Could you check a few things on this model? Use its own coordinates, in mm. A direction names the side the tool comes from. Coordinates: 2 decimals unless noted, no trailing zeros. Write each loop counter-clockwise with the first axis right and the second up, starting at its lowest first coordinate (ties: lowest second). Pieces come first, ordered by that corner, then holes.
```python
from build123d import *

# Parameters (mm, degrees)
F0_W     = 88.9
F0_H     = 63.5
F0_W_2   = 64.688936
F0_H_2   = 39.437553
F1_DEPTH = 25.4
F2_W     = 64.972658
F2_H     = 38.870107
F3_DEPTH = 7.62
F5_DEPTH = 19.05
F7_DEPTH = 19.05


with BuildPart() as f1:
    # F0 (on Top) → F1 (new body)
    with BuildSketch(Plane.XY):
        with Locations((-7.991541, 0.256701)):
            Rectangle(F0_W, F0_H)
        with Locations((-8.937288, 0.425585)):
            Rectangle(F0_W_2, F0_H_2, mode=Mode.SUBTRACT)
    extrude(amount=F1_DEPTH)

    # F2 (on Top) → F3 (join)
    with BuildSketch(Plane.XY):
        with Locations((-9.079149, 0.425584)):
            Rectangle(F2_W, F2_H)
    extrude(amount=F3_DEPTH)

    # F4 (on Top) → F5 (join)
    with BuildSketch(Plane.XY):
        Polygon((-14.895479, 10.781489), (-34.756117, 10.781489), (-34.756117, 2.269787), (-28.797926, 2.269787), (-28.797926, -13.902447), (-21.421118, -13.902447), (-21.421118, 2.269787), (-14.895479, 2.269787), align=None)
    extrude(amount=F5_DEPTH)

    # F6 (on Top) → F7 (join)
    with BuildSketch(Plane.XY):
        Polygon((2.127926, 10.497767), (-3.830266, 10.497767), (-3.830266, -13.335001), (14.895479, -13.335001), (14.895479, -6.241915), (2.127926, -6.241915), align=None)
    extrude(amount=F7_DEPTH)


solid = f1.part
```
Item 1: I want a section at D-D, the plane z = 23.25. List the corners of the cut face in (x, y) for me.
Item 2: I want a section at B-B, the plane x = -20.5. List the corners of the cut face in (y, z) for me.
Item 3: Which directions (+Z, -Z, +X, -X, +Y, -Y) give clear straight access to the entire face, cutting with the end or side of a thin tool? Please do faces 1 (the flat face through (-52.442, 0, 13)), 2 (the flat face through (5, -13.335, 13)), 3 (the flat face through (-9, -19.293, 13)).
Item 4: I want a section at A-A, the plane z = 13.5. List the corners of the cut face in (x, y) for me (3 decimals), then the cut area to 3 significant figures.
Item 5: If we mould it in two halves opening along Y, with no side actions, what happens to faces 4 (the flat face through (-9, -31.493, 13)), 5 (the flat face through (-9, 1, 0)), 6 (the flat face through (-28.798, -6, 13))? For each: released by +Y, released by -Y, zero draft, split by the parting line, or undercut.
Item 6: If I drill on line 1 along Y through (x, z) = (-23.5, 2.25); line 2 along X through (y, z) = (7, 9.5); line 3 along Y through (x, z) = (-29, 13), over which ranges is the centre line in solid material (lowest first)?
Item 7: Will these pins go through, and if not, where does the flat tip stop? pin 1 Ø3 at (x, y) = (-15, 8.5) entering from +Z; pin 2 Ø1 at (x, y) = (-40.5, 8.5) entering from +Z.
Item 8: I want a section at C-C, the plane y = 9. List the corners of the cut face in (x, z) for me, then the cut area to 3 significant figures.
Taken from the geometry:
1. outline: (-52.44, -31.49) - (36.46, -31.49) - (36.46, 32.01) - (-52.44, 32.01) - close; hole (-41.28, -19.29) - (23.41, -19.29) - (23.41, 20.14) - (-41.28, 20.14) - close
2. outline: (-31.49, 0) - (-19.29, 0) - (-19.29, 25.4) - (-31.49, 25.4) - close; (-19.01, 0) - (19.86, 0) - (19.86, 7.62) - (10.78, 7.62) - (10.78, 19.05) - (2.27, 19.05) - (2.27, 7.62) - (-19.01, 7.62) - close; (20.14, 0) - (32.01, 0) - (32.01, 25.4) - (20.14, 25.4) - close
3. face 1: +Z, -Z, -X, +Y, -Y
3. face 2: +Z
3. face 3: +Z, -Z
4. outline: (-52.442, -31.493) - (36.458, -31.493) - (36.458, 32.007) - (-52.442, 32.007) - close; (-34.756, 2.27) - (-28.798, 2.27) - (-28.798, -13.902) - (-21.421, -13.902) - (-21.421, 2.27) - (-14.895, 2.27) - (-14.895, 10.781) - (-34.756, 10.781) - close; (-3.83, -13.335) - (14.895, -13.335) - (14.895, -6.242) - (2.128, -6.242) - (2.128, 10.498) - (-3.83, 10.498) - close; hole (-41.282, -19.293) - (23.407, -19.293) - (23.407, 20.144) - (-41.282, 20.144) - close
4. area: 3,610 mm2
5. face 4: released by -Y
5. face 5: zero draft
5. face 6: undercut
6. line 1: y = -31.49 to -19.29, -19.01 to 19.86, 20.14 to 32.01
6. line 2: x = -52.44 to -41.28, -34.76 to -14.9, -3.83 to 2.13, 23.41 to 36.46
6. line 3: y = -31.49 to -19.29, 2.27 to 10.78, 20.14 to 32.01
7. pin 1: stops at z = 19.05
7. pin 2: stops at z = 7.62
8. outline: (-52.44, 0) - (36.46, 0) - (36.46, 25.4) - (23.41, 25.4) - (23.41, 7.62) - (2.13, 7.62) - (2.13, 19.05) - (-3.83, 19.05) - (-3.83, 7.62) - (-14.9, 7.62) - (-14.9, 19.05) - (-34.76, 19.05) - (-34.76, 7.62) - (-41.28, 7.62) - (-41.28, 25.4) - (-52.44, 25.4) - close
8. area: 1,400 mm2
